Geometry: final body of the model. Coordinates: model frame, mm. Give positions to 0.01 mm unless a question says otherwise; leave off trailing zeros. Loops run counter-clockwise (first coordinate to the right, second up) from the corner with the lowest first, then second, coordinate; pieces in that order, holes last.
1. Section C-C, the plane x = 68.5. Output: boundary loops of the cut face in (y, z) (3 decimals), then the cut area to 3 significant figures.
2. Section B-B, the plane y = 0.5. State how many separate pieces and enclosed holes the cut face has, then the cut area to 3 significant figures.
3. Material intervals for line 1 along X through (y, z) = (0.9, -130) (3 decimals), sorted ascending.
4. Draft query along X for faces 1 (the face through (-4.82, 1.57, -105.95)), 2 (the face through (-5.786, 1.565, -33.594)), 3 (the face through (69, 0, -74)). Return one class per face: +X half, -X half, draft (parallel to the pull), parting line (faces both ways), or undercut.
5. Section A-A, the plane x = 15. Output: boundary loops of the cut face in (y, z) (3 decimals).
6. First-contact query: P1, Ø9, axis at x = 145.21, z = -36.39, coming from the -Y side; P2, Ø1, axis at x = 69.5, y = 2, coming from the -Z side. Flat tips, straight axial feed; report the tip coordinate or a pass-through.
from build123d import *

# Parameters (mm, degrees)
SKETCH1_R           = 3.175
SKETCH1_R_2         = 2.794
BOSS_EXTRUDE3_DEPTH = 3.175


with BuildPart() as part:
    # Sketch1 → Boss-Extrude3 (new body)
    with BuildSketch(Plane(origin=(0, 0, 0), x_dir=(1, 0, 0), z_dir=(0, 1, 0))):
        Polygon((0, 0), (64.775, 0), (64.775, 20), (74.775, 20), (74.775, 0), (155.5, 0), (155.5, 145), (139.55, 145), (74.775, 145), (74.775, 125), (64.775, 125), (64.775, 130), (64.775, 145), (0, 145), (-15.95, 145), (-15.95, 0), align=None)
        with Locations(Location((15, 130, 0), (0, 0, 270))):
            Circle(SKETCH1_R, mode=Mode.SUBTRACT)
        with Locations(Location((124.55, 130, 0), (0, 0, 90))):
            Circle(SKETCH1_R, mode=Mode.SUBTRACT)
        with Locations(Location((15, 15, 0), (0, 0, 90))):
            Circle(SKETCH1_R, mode=Mode.SUBTRACT)
        with Locations(Location((124.55, 15, 0), (0, 0, 270))):
            Circle(SKETCH1_R, mode=Mode.SUBTRACT)
        with Locations(Location((-5.663, 134.0145, 0), (0, 0, 270))):
            Circle(SKETCH1_R_2, mode=Mode.SUBTRACT)
        with Locations(Location((-5.663, 108.6145, 0), (0, 0, 270))):
            Circle(SKETCH1_R_2, mode=Mode.SUBTRACT)
        with Locations(Location((145.213, 134.0145, 0), (0, 0, 90))):
            Circle(SKETCH1_R_2, mode=Mode.SUBTRACT)
        with Locations(Location((145.213, 108.6145, 0), (0, 0, 90))):
            Circle(SKETCH1_R_2, mode=Mode.SUBTRACT)
        with Locations(Location((-5.663, 36.3855, 0), (0, 0, 90))):
            Circle(SKETCH1_R_2, mode=Mode.SUBTRACT)
        with Locations(Location((-5.663, 10.9855, 0), (0, 0, 90))):
            Circle(SKETCH1_R_2, mode=Mode.SUBTRACT)
        with Locations(Location((145.213, 10.9855, 0), (0, 0, 270))):
            Circle(SKETCH1_R_2, mode=Mode.SUBTRACT)
        with Locations(Location((145.213, 36.3855, 0), (0, 0, 270))):
            Circle(SKETCH1_R_2, mode=Mode.SUBTRACT)
    extrude(amount=BOSS_EXTRUDE3_DEPTH)


solid = part.part
Answers below:
1. outline: (0, -125) - (3.175, -125) - (3.175, -20) - (0, -20) - close
1. area: 333 mm2
2. separate pieces: 1
2. enclosed holes: 12
2. area: 24,100 mm2
3. line 1: x = -15.95 to 11.825, 18.175 to 64.775, 74.775 to 121.375, 127.725 to 155.5
4. face 1: undercut
4. face 2: undercut
4. face 3: draft
5. outline: (0, -145) - (3.175, -145) - (3.175, -133.175) - (0, -133.175) - close; (0, -126.825) - (3.175, -126.825) - (3.175, -18.175) - (0, -18.175) - close; (0, -11.825) - (3.175, -11.825) - (3.175, 0) - (0, 0) - close
6. P1: stops at y = 0
6. P2: stops at z = -125
